Answer from the drawing. Dimensions are ordinates in mm from the lowest x, y and z of the part. Give positions to 0.01 mm unless a question says otherwise; leave off trailing zeros. Loops run counter-clockwise (first coordinate to the right, second up) from the corner with the lowest first, then second, coordinate; pieces in that order, holes last. Notation, with made-up numbers: (27.25, -13.5) - (32.25, -13.5) arc R19 ccw to (32.25, 21.5) - close; hole circle Ø2 at (-24, -9). An arc over 180 degrees is marked (long way). Answer as CSV lines item,"result". Start each with the question number.
1) A flat-ended cylindrical pin translates along its axis: pin 1 (1.5 mm diameter, centred on y = 8.5, z = 23, fed in from -X). Find the tip coordinate at first contact, or state that the pin passes through.
2) A cutting plane is placed at A-A (y = 17). Determine the outline of the cut face in (x, z) (1 decimal).
3) A cutting plane is placed at B-B (x = 896). Determine the outline of the cut face in (y, z), and give its area (3 significant figures).
4) Find the intervals of material crossed by line 1 along Z through (x, y) = (71.5, 8); line 2 along X through (y, z) = (19.5, 59); line 3 along X through (y, z) = (10, 32) (1 decimal), in increasing order.
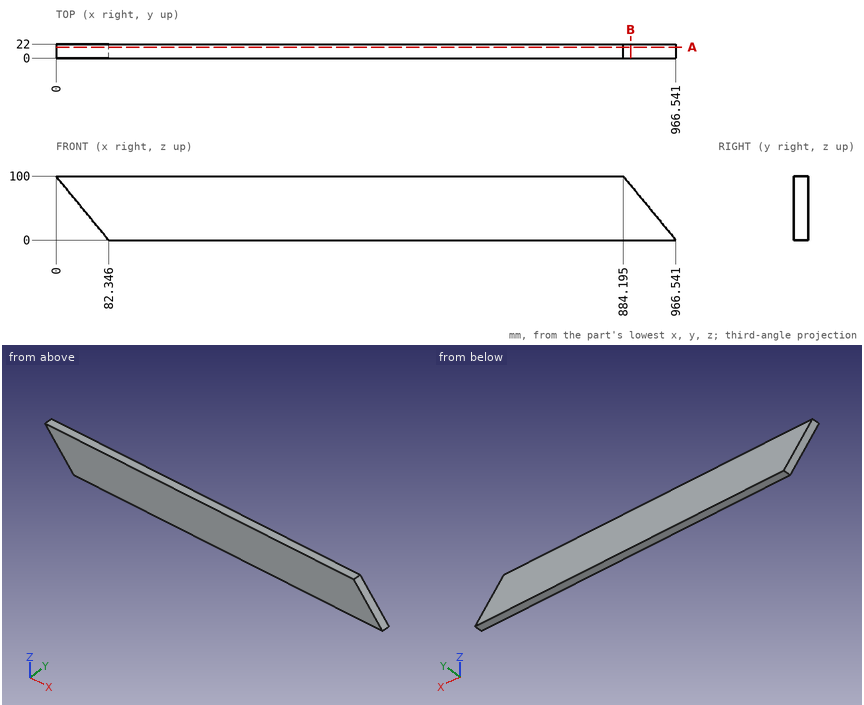
Ans:
1,pin 1,"x = 62.79"
2,outline,"(0, 100) - (82.3, 0) - (966.5, 0) - (884.2, 100) - close"
3,outline,"(0, 0) - (22, 0) - (22, 85.66) - (0, 85.66) - close"
3,area,"1,880 mm2"
4,line 1,"13.17 to 100"
4,line 2,"33.76 to 917.96"
4,line 3,"56 to 940.2"
